Design review of the part shown in the three views and the two pictorial views. Dimensions are in mm from the part's minimum x, y and z. Give positions to 0.01 mm unless a question says otherwise; leave off trailing zeros. Order: outer loops, then holes, each group sorted by start corner. A loop starts at its lowest first (then second) coordinate and runs counter-clockwise, first axis right, second up.
Item 1: Consider section B-B (z = 20). Give the boundary of the cut face in (x, y), plus the area to 3 significant figures.
Item 2: Consider section A-A (x = 7.5). Give the boundary of the cut face in (y, z), plus the area to 3 significant figures.
Item 3: For probe 1 along X at (y, z) = (0.7, 20); probe 2 along Z at (x, y) = (6.5, 1); probe 3 along X at (y, z) = (1.2, 19.5), list the stretches that pass through material, from the lowest coordinate up.
Item 4: Consider section C-C (y = 1.05). Give the boundary of the cut face in (x, z).
Item 5: The part is to be moulded in two halves that separate along Y. For the marked faces 1 and 2, say which applies: released by +Y, released by -Y, zero draft, split by the parting line, or undercut.
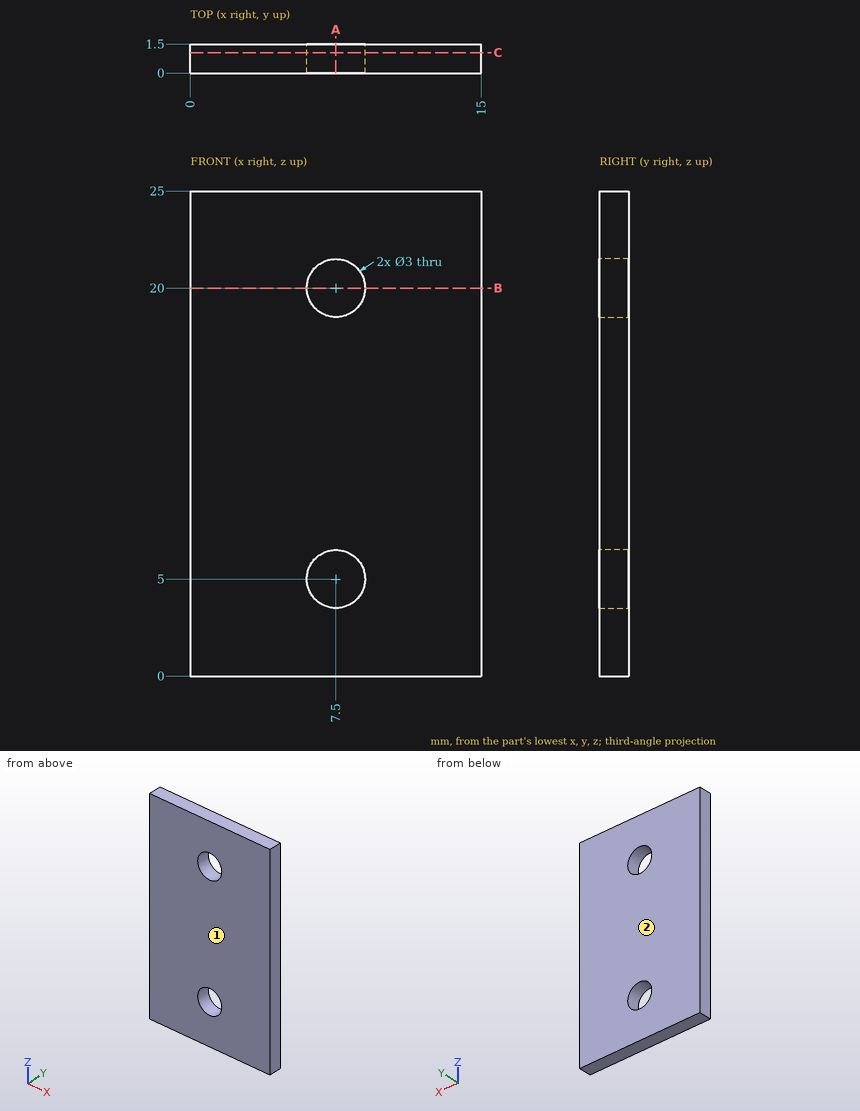
Resolved:
1. outline: (0, 0) - (6, 0) - (6, 1.5) - (0, 1.5) - close; (9, 0) - (15, 0) - (15, 1.5) - (9, 1.5) - close
1. area: 18.0 mm2
2. outline: (0, 0) - (1.5, 0) - (1.5, 3.5) - (0, 3.5) - close; (0, 6.5) - (1.5, 6.5) - (1.5, 18.5) - (0, 18.5) - close; (0, 21.5) - (1.5, 21.5) - (1.5, 25) - (0, 25) - close
2. area: 28.5 mm2
3. probe 1: x = 0 to 6, 9 to 15
3. probe 2: z = 0 to 3.88, 6.12 to 18.88, 21.12 to 25
3. probe 3: x = 0 to 6.09, 8.91 to 15
4. outline: (0, 0) - (15, 0) - (15, 25) - (0, 25) - close; hole circle Ø3 at (7.5, 5); hole circle Ø3 at (7.5, 20)
5. face 1: released by -Y
5. face 2: released by +Y
